Verification items for the finished model (mm, model axes). A direction names the side the tool comes from. Give positions to 0.01 mm unless a question says otherwise; leave off trailing zeros. Write each loop counter-clockwise with the first axis right and the second up, starting at its lowest first coordinate (ties: lowest second). Pieces come first, ordered by that corner, then holes. Notation, with made-up numbers: (49.25, -2.5) -> (86.25, -2.5) arc R15 ccw to (86.25, 15.5) -> close; hole circle Ø9 at (57.25, -31.75). An arc over 180 degrees is marked (long way). Answer as CSV lines item,"result". Start each with the question number.
1) Tool access check on faces 5 (the flat face through (142.922, 214.563, 9.86)), 6 (the cylindrical face through (-73.25, 4.93, 7.05)). Record the directions out of +Z, -Z, +X, -X, +Y, -Y that give a thin tool (end or side, any length) a straight path to the whole face; none if there is none.
2) Sectioned sample at D-D on z = 10. Give the number of separate pieces and of enclosed holes in the cut face, and give its area (3 significant figures).
3) Sectioned sample at C-C on x = 15. Record the cut outline in (y, z).
4) Gauge pin test, flat ends, axial feed: pin 1 Ø21.5 at (x, y) = (107.05, 47.78) entering from -Z; pin 2 Ø2 at (y, z) = (39.5, 7.5) entering from +X; pin 3 Ø3 at (y, z) = (198.5, 17) entering from +X; pin 4 Ø12 at (x, y) = (-30, 164) entering from +Z. Record the tip position at first contact, or that the pin passes through.
5) Sectioned sample at B-B on y = 138. Record the cut outline in (x, z).
6) Material ranges on L1, parallel to Y at x = 114, z = 18; L2, parallel to X at y = 168, z = 8.75; L3, parallel to X at y = 239.75, z = 10, recorded low to high.
7) Mould release check, pull along X, two halves, no side actions. Record for faces 1 (the cylindrical face through (170.07, 148.034, 9.479)), 2 (the flat face through (20.94, 138.24, -1.97)), 3 (the flat face through (-21.082, 138.042, -5.972)), 4 (the flat face through (-141.07, 28.76, 9.86)): released by +X, released by -X, zero draft, split by the parting line, or undercut.
8) Sectioned sample at A-A on x = -56. Record the cut outline in (y, z).
Autodesk Inventor part; units mm, degrees
ref_plane "Work Plane1" through (0, 0, 0) normal (0, 0, -1) x (-1, 0, 0)
ref_plane "Work Plane3" through (0, 0, -4) normal (0, 0, -1) x (-1, 0, 0)
ref_plane "YZ Plane" through (0, 0, 0) normal (1, 0, 0) x (0, 1, 0)
sketch "Sketch1" plane through (0, 0, 0) normal (0, 0, 1) x (1, 0, 0)
  line L0 (0, 0) -> (-116.4534, 0)
  line L1 (-175, 47) -> (-175, 187)
  line L2 (-118.5466, 245) -> (0, 245)
  line L3 (0, 245) -> (0, 0) construction
  line L4 (-118.5466, 235) -> (-9, 235)
  line L5 (-9, 10) -> (-116.4534, 10)
  line L6 (-165, 47) -> (-165, 187)
  line L7 (0, 0) -> (123.5466, 0)
  line L8 (175, 53.5466) -> (175, 193.5466)
  line L9 (121.4534, 245) -> (0, 245)
  line L10 (121.4534, 235) -> (9, 235)
  line L11 (9, 10) -> (123.5466, 10)
  line L12 (165, 53.5466) -> (165, 193.5466)
  line L13 (-9, 235) -> (9, 235)
  line L14 (-9, 10) -> (9, 10)
  line L15 (-175, 187) -> (-118.5466, 245)
  line L16 (-175, 47) -> (-116.4534, 0)
  line L17 (121.4534, 245) -> (175, 193.5466)
  line L18 (175, 53.5466) -> (123.5466, 0)
  line L19 (-175, 47) -> (-165, 47)
  line L20 (-116.4534, 10) -> (-116.4534, 0)
  line L21 (-118.5466, 245) -> (-118.5466, 235)
  line L22 (-175, 187) -> (-165, 187)
  line L23 (-118.5466, 235) -> (-165, 187)
  line L24 (-165, 47) -> (-116.4534, 10)
  line L25 (121.4534, 245) -> (121.4534, 235)
  line L26 (175, 193.5466) -> (165, 193.5466)
  line L27 (121.4534, 235) -> (165, 193.5466)
  line L28 (175, 53.5466) -> (165, 53.5466)
  line L29 (123.5466, 0) -> (123.5466, 10)
  line L30 (123.5466, 10) -> (165, 53.5466)
  point P0 (-175, 245)
  point P1 (-175, 0)
  point P2 (-165, 235)
  point P3 (-165, 10)
  point P4 (175, 245)
  point P5 (175, 0)
  point P6 (165, 235)
  point P7 (165, 10)
  dimension "d0" = 245
  dimension "d1" = 175
  dimension "d4" = 10
  dimension "d7" = 240
  dimension "d9" = 240
  dimension "d10" = 140
  dimension "d12" = 136.142
  dimension "d13" = 133.589
  dimension "d14" = 52.687
  dimension "d15" = 44.062
  dimension "d16" = 44.226
  dimension "d17" = 51.243
  dimension "d18" = 10
  dimension "d19" = 53.5466
  dimension "d20" = 175
  dimension "d21" = 0
  dimension "d22" = 0
  dimension "d23" = 10
  dimension "d24" = 41.4534
  dimension "d25" = 10
  dimension "d26" = 183.5465
  dimension "d27" = 166
  dimension "d28" = 166
extrude "Extrusion1" add sketch "Sketch1" along normal blind 20 contours L0 L20 L5 L14 L11 L29 L7 | L16 L19 L24 L20 | L29 L30 L28 L18 | L1 L22 L6 L19 | L28 L12 L26 L8 | L15 L21 L23 L22 | L26 L27 L25 L17 | L2 L9 L25 L10 L13 L4 L21
ref_plane "Work Plane1" through (0, 0, 0) normal (0, 0, -1) x (-1, 0, 0)
sketch "Sketch2" plane through (0, 0, 0) normal (0, 0, -1) x (-1, 0, 0)
  line L0 (-123.5466, 0) -> (-175, 53.5466)
  line L1 (-175, 53.5466) -> (-175, 0)
  line L2 (-175, 0) -> (-123.5466, 0)
  line L3 (175, 187) -> (175, 47)
  line L4 (175, 47) -> (175, 0)
  line L5 (116.4534, 0) -> (-123.5466, 0)
  line L6 (175, 0) -> (116.4534, 0)
  line L7 (-121.4534, 245) -> (118.5466, 245)
  line L8 (118.5466, 245) -> (175, 245)
  line L9 (175, 245) -> (175, 187)
  line L10 (-121.4534, 245) -> (-175, 245)
  line L11 (-175, 245) -> (-175, 193.5466)
  line L12 (-175, 193.5466) -> (-121.4534, 245)
  line L13 (-160.5333, -20.6513) -> (189.4198, 224.4003)
  line L14 (-189.2819, 20.4027) -> (160.7181, 265.4027)
  circle A0 centre (101, 198.51) radius 12
  circle A1 centre (56, 161.7) radius 12.5
  circle A2 centre (-107.0481, 47.7774) radius 12
  circle A3 centre (-62.0481, 79.2774) radius 12.5
  line L15 (160.7181, 265.4027) -> (189.4198, 224.4003)
  line L16 (-189.238, 20.3554) -> (-160.5333, -20.6513)
  line L17 (118.5466, 245) -> (175, 187)
  point P0 (0, 0)
  point P1 (159.1963, 203.2366)
  point P2 (123.8247, 239.5773)
  point P3 (-161.7026, 39.7082)
  point P4 (-126.5613, 3.1373)
  dimension "d32" = 45
  dimension "d33" = 45
  dimension "d34" = 24
  dimension "d35" = 25
  dimension "d36" = 24
  dimension "d37" = 25
  dimension "d38" = 45
extrude "Extrusion2" add sketch "Sketch2" along normal blind 4 contours L0 L14 L17 L13
ref_plane "Work Plane3" through (0, 0, -4) normal (0, 0, -1) x (-1, 0, 0)
sketch "Sketch4" plane through (0, 0, -4) normal (0, 0, -1) x (-1, 0, 0)
  line L0 (175, 47) -> (116.4534, 0)
  line L1 (116.4534, 0) -> (175, 0)
  line L2 (175, 0) -> (175, 47)
  line L3 (175, 187) -> (175, 245)
  line L4 (118.5466, 245) -> (175, 187)
  line L5 (175, 245) -> (118.5466, 245)
  line L6 (-175, 193.5466) -> (-121.4534, 245)
  line L7 (-121.4534, 245) -> (-175, 245)
  line L8 (-175, 245) -> (-175, 193.5466)
  line L9 (-123.5466, 0) -> (-175, 0)
  line L10 (-175, 0) -> (-175, 53.5466)
  line L11 (175, 0) -> (-175, 245)
  line L12 (160.906, -20.1342) -> (-189.094, 224.8658)
  line L13 (189.2349, 20.3356) -> (-160.7651, 265.3356)
  line L14 (160.906, -20.1342) -> (189.2349, 20.3356)
  line L15 (-189.094, 224.8658) -> (-160.7651, 265.3356)
  circle A0 centre (105.3249, 48.7726) radius 12
  circle A1 centre (60.3249, 80.2726) radius 12.5
  circle A2 centre (-106.4463, 197.0124) radius 12.5
  circle A3 centre (-61.4463, 165.5124) radius 12.5
  point P0 (0, 0)
  point P1 (163.8873, 38.0789)
  point P2 (-125.7779, 240.8446)
  point P3 (-162.0833, 205.9583)
  point P4 (123.7616, 5.8669)
  dimension "d46" = 24.577
  dimension "d47" = 24.8227
  dimension "d48" = 45
  dimension "d50" = 45
  dimension "d51" = 45
  dimension "d52" = 45
  dimension "d55" = 25
  dimension "d56" = 25
  dimension "d59" = 25
  dimension "d60" = 24
extrude "Extrusion3" add sketch "Sketch4" along normal blind 4 contours L0 L11 A0 A1 A3 A2 L6 L13 | L0 L12 L6 L11 A2 A3 A1 A0
sketch "Sketch5" plane through (-118.5466, 245, 0) normal (0, 1, 0) x (1, 0, 0)
  line L0 (240, 0) -> (0, 0)
  line L1 (0, 0) -> (0, -20)
  point P0 (118.5466, 0)
  point P1 (48, -10)
  point P2 (96, -10)
  point P3 (144, -10)
  point P4 (192, -10)
  dimension "d70" = 10
  dimension "d71" = 48
  dimension "d72" = 48
  dimension "d73" = 48
  dimension "d74" = 48
hole "Hole1" at (-70.5466, 245, 10) at (-22.5466, 245, 10) at (25.4534, 245, 10) at (73.4534, 245, 10) direction (0, -1, 0) diameter 8 end through all
sketch "Sketch6" plane through (-175, 47, 0) normal (-1, 0, 0) x (0, 0, 1)
  line L0 (0, 0) -> (20, 0)
  line L1 (0, 140) -> (0, 0)
  point P0 (0, -47)
  point P1 (10, 35)
  point P2 (10, 70)
  point P3 (10, 105)
  dimension "d82" = 35
  dimension "d83" = 10
  dimension "d84" = 35
  dimension "d85" = 35
hole "Hole2" at (-175, 82, 10) at (-175, 117, 10) at (-175, 152, 10) direction (1, 0, 0) diameter 8 end through all
properties part number "New Chassis"
Ans:
1,face 5,"+Z"
1,face 6,"+Y, -Y"
2,separate pieces,"14"
2,enclosed holes,"0"
2,area,"8,430 mm²"
3,outline,"(0, 0) -> (10, 0) -> (10, 20) -> (0, 20) -> close; (81.26, -4) -> (103, -4) -> (103, -8) -> (163.3, -8) -> (163.3, -4) -> (142.4, -4) -> (142.4, 0) -> (81.26, 0) -> close; (235, 0) -> (245, 0) -> (245, 20) -> (235, 20) -> close"
4,pin 1,"passes through"
4,pin 2,"stops at x = 162.46"
4,pin 3,"stops at x = 171.41"
4,pin 4,"stops at z = 0"
5,outline,"(-175, 0) -> (-165, 0) -> (-165, 20) -> (-175, 20) -> close; (-66.03, -4) -> (-21.14, -4) -> (-21.14, -8) -> (65, -8) -> (65, -4) -> (21.29, -4) -> (21.29, 0) -> (-66.03, 0) -> close; (165, 0) -> (175, 0) -> (175, 20) -> (165, 20) -> close"
6,L1,"y = 0 to 10, 235 to 245"
6,L2,"x = -175 to -165, 165 to 175"
6,L3,"x = -123.66 to -74.55, -66.55 to -26.55, -18.55 to 21.45, 29.45 to 69.45, 77.45 to 126.92"
7,face 1,"zero draft"
7,face 2,"released by +X"
7,face 3,"released by -X"
7,face 4,"undercut"
8,outline,"(0, 0) -> (10, 0) -> (10, 20) -> (0, 20) -> close; (53.3, -8) -> (68.54, -8) -> (68.54, -4) -> (53.3, -4) -> close; (92, -8) -> (113.6, -8) -> (113.6, -4) -> (92, -4) -> close; (130.97, -4) -> (149.2, -4) -> (149.2, 0) -> (130.97, 0) -> close; (174.2, -4) -> (192.1, -4) -> (192.1, 0) -> (174.2, 0) -> close; (235, 0) -> (245, 0) -> (245, 20) -> (235, 20) -> close"
